Geometry: final body of the model. Coordinates: model frame, mm. A direction names the side the tool comes from. Give positions to 0.01 mm unless a question says otherwise; leave off trailing zeros. Write each loop counter-clockwise with the first axis right and the second up, starting at its lowest first coordinate (ties: lowest second). Pieces come first, ordered by that corner, then holes. Notation, with made-up numbers: (1, 67.5) -> (16, 67.5) arc R20 ccw to (16, 102.5) -> close; hole circle Ø10 at (35.5, -19.5). An arc over 180 degrees is marked (long way). Answer as a JSON object with one key per item and string values. Group by question number.
(1) Section query C-C on y = -21. Output: boundary loops of the cut face in (x, z).
(2) Draft query along Z for faces 1 (the face through (-4.686, -7.951, 35.694)), 2 (the face through (-10.154, -23.824, 77.336)), 3 (the face through (81, -23.5, 21)). Return one class per face: +Z half, -Z half, draft (parallel to the pull), parting line (faces both ways), or undercut.
(3) Set-up query: faces 4 (the face through (15.8, -4.5, -29.2)), 5 (the face through (-11.195, -50.548, 85.268)), 6 (the face through (74, -13, -31)). Return all of +Z, -Z, +X, -X, +Y, -Y with unobstructed straight access to the full face (end or side cutting, diameter ignored); none if empty.
(4) Section query B-B on x = 0. State how many separate pieces and enclosed holes the cut face has, plus the area to 3 significant figures.
(5) Contact query for flat-ended pins moving along their axis: pin 1 Ø4 at (x, z) = (-39.5, -50.5) entering from -Y; pin 2 Ø3 at (y, z) = (-36, -55.5) entering from +X; pin 3 Ø1.5 at (y, z) = (-15, 26.5) entering from -X; pin 4 Ø8 at (x, z) = (33.59, -46.24) entering from -Y. Output: stop coordinate, or through.
(6) Material intervals for probe 1 along Z at (x, y) = (0, -13.5); probe 2 along Z at (x, y) = (0, -50); probe 3 along Y at (x, z) = (-14, 39.5), sorted ascending.
(7) Section query D-D on x = -58. Output: boundary loops of the cut face in (y, z), plus the area to 3 significant figures.
from build123d import *

# Parameters (mm, degrees)
F2_R     = 6.5
F3_DEPTH = 5.5
F4_DEPTH = 77.001


with BuildPart() as f1:
    # F0 (on Top) → F1 (revolve)
    with BuildSketch(Plane.XY):
        Polygon((86, -29), (86, -71.5), (91.5, -71.5), (91.5, -23.5), (83.5, -23.5), (83.5, -13), (79.5, -13), (79.5, -11.5), (36, -11.5), (36, -4.5), (33.05, -4.5), (33.05, 5.5), (0, 5.5), (0, 0), (27.55, 0), (27.55, -10), (30.5, -10), (30.5, -17), (74, -17), (74, -18.5), (78, -18.5), (78, -29), align=None)
    revolve(axis=Axis((0, 2.75, 0), (0, -1, 0)))

    # F2 (on face) → F3 (cut, through all)
    with BuildSketch(Plane(origin=(0, -11.5, 0), x_dir=(-1, 0, 0), z_dir=(0, 1, 0))):
        with Locations((0, 57.15)):
            Circle(F2_R)
        with Locations((-54.3528799063, 17.6603212285)):
            Circle(F2_R)
        with Locations((-33.5919271685, -46.2353212285)):
            Circle(F2_R)
        with Locations((33.5919271685, -46.2353212285)):
            Circle(F2_R)
        with Locations((54.3528799063, 17.6603212285)):
            Circle(F2_R)
    extrude(amount=-F3_DEPTH, mode=Mode.SUBTRACT)

    # F4 (cut, through all): a face of the model
    f4_faces = [f1.faces().sort_by_distance(p)[0] for p in [
        (0, 5.5, 0),
    ]]
    extrude(f4_faces, amount=-F4_DEPTH, mode=Mode.SUBTRACT)


solid = f1.part
Answer list:
{
 "1": {"outline": "circle Ø167 at (0, 0); hole circle Ø156 at (0, 0)"},
 "2": {"face 1": "parting line", "face 2": "undercut", "face 3": "draft"},
 "3": {"face 4": "+Z, -Z, +X, -X, +Y", "face 5": "-Y", "face 6": "+Y"},
 "4": {"separate pieces": "3", "enclosed holes": "0", "area": "1,210 mm2"},
 "5": {"pin 1": "y = -17", "pin 2": "x = 73.87", "pin 3": "x = -79.43", "pin 4": "through"},
 "6": {"probe 1": "-83.5 to -33.05, 33.05 to 50.65, 63.65 to 83.5", "probe 2": "-91.5 to -86, 86 to 91.5", "probe 3": "-17 to -11.5"},
 "7": {"outline": "(-71.5, -70.77) -> (-23.5, -70.77) -> (-23.5, -60.07) -> (-13, -60.07) -> (-13, -54.37) -> (-11.5, -54.37) -> (-11.5, 12.28) -> (-17, 12.28) -> (-17, -45.96) -> (-18.5, -45.96) -> (-18.5, -52.15) -> (-29, -52.15) -> (-29, -63.5) -> (-71.5, -63.5) -> close; (-71.5, 63.5) -> (-29, 63.5) -> (-29, 52.15) -> (-18.5, 52.15) -> (-18.5, 45.96) -> (-17, 45.96) -> (-17, 23.04) -> (-11.5, 23.04) -> (-11.5, 54.37) -> (-13, 54.37) -> (-13, 60.07) -> (-23.5, 60.07) -> (-23.5, 70.77) -> (-71.5, 70.77) -> close", "area": "1,530 mm2"}
}
